For this review, take the finished solid that the model builds, in its own axes (mm). Round coordinates to 2 decimals unless told otherwise and drop trailing zeros. Order: outer loops, then holes, each group sorted by start corner. A loop starts at its lowest first (then second) coordinate and runs counter-clockwise, first axis right, second up. Notation, with made-up numbers: M -9.75,-11 L 45.25,-11 A25 cw 45.25,21 Z; hole C -23,-34.75 d11. An arc over 180 degrees is marked long. Put each result on its own line as item: value.
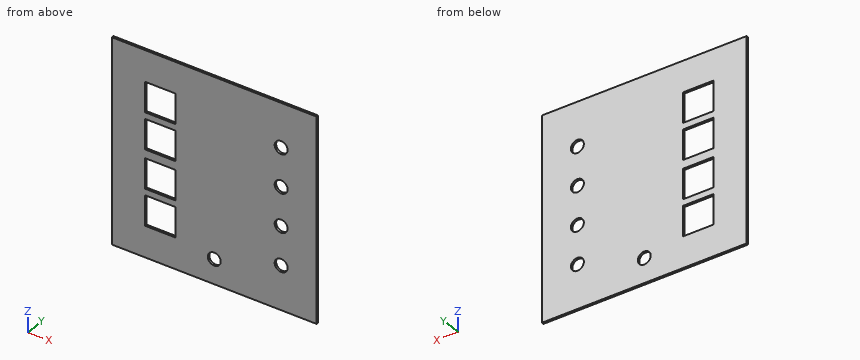
from build123d import *

# Parameters (mm, degrees)
SKETCH1_W           = 95
SKETCH1_H           = 95
BOSS_EXTRUDE1_DEPTH = 1
SKETCH2_R           = 3
SKETCH2_W           = 14
SKETCH2_H           = 14
CUT_EXTRUDE1_DEPTH  = 1


with BuildPart() as part:
    # Sketch1 → Boss-Extrude1 (new body)
    with BuildSketch(Plane(origin=(0, 0, 0), x_dir=(1, 0, 0), z_dir=(0, 1, 0))):
        with Locations((47.5, 47.5)):
            Rectangle(SKETCH1_W, SKETCH1_H)
    extrude(amount=BOSS_EXTRUDE1_DEPTH)

    # Sketch2 → Cut-Extrude1 (cut)
    with BuildSketch(Plane(origin=(0, 1, 0), x_dir=(1, 0, 0), z_dir=(0, 1, 0))):
        with Locations(Location((47.5, 83.5, 0), (0, 0, 270))):
            Circle(SKETCH2_R)
        with Locations(Location((78.5, 74.5, 0), (0, 0, 270))):
            Circle(SKETCH2_R)
        with Locations(Location((78.5, 56.5, 0), (0, 0, 270))):
            Circle(SKETCH2_R)
        with Locations(Location((78.5, 38.5, 0), (0, 0, 90))):
            Circle(SKETCH2_R)
        with Locations(Location((78.5, 20.5, 0), (0, 0, 90))):
            Circle(SKETCH2_R)
        with Locations((22.5, 56.5)):
            Rectangle(SKETCH2_W, SKETCH2_H)
        with Locations((22.5, 73.5)):
            Rectangle(SKETCH2_W, SKETCH2_H)
        with Locations((22.5, 21.5)):
            Rectangle(SKETCH2_W, SKETCH2_H)
        with Locations((22.5, 38.5)):
            Rectangle(SKETCH2_W, SKETCH2_H)
    extrude(amount=-CUT_EXTRUDE1_DEPTH, mode=Mode.SUBTRACT)


solid = part.part
(1) Add section B-B on x = 47.5. Give the boundary of the cut face in (y, z), then the cut area to 3 significant figures.
A:
outline: M 0,-95 L 1,-95 L 1,-86.5 L 0,-86.5 Z; M 0,-80.5 L 1,-80.5 L 1,0 L 0,0 Z
area: 89.0 mm2
(2) Add section A-A on z = -83.5. Give the boundary of the cut face in (x, y), then the cut area to 3 significant figures.
A:
outline: M 0,0 L 44.5,0 L 44.5,1 L 0,1 Z; M 50.5,0 L 95,0 L 95,1 L 50.5,1 Z
area: 89.0 mm2
(3) Add section C-C on z = -56.5. Give the boundary of the cut face in (x, y), then the cut area to 3 significant figures.
A:
outline: M 0,0 L 15.5,0 L 15.5,1 L 0,1 Z; M 29.5,0 L 75.5,0 L 75.5,1 L 29.5,1 Z; M 81.5,0 L 95,0 L 95,1 L 81.5,1 Z
area: 75.0 mm2
(4) Add section D-D on y = 0.6. State how many separate pieces and enclosed holes the cut face has, then the cut area to 3 significant figures.
A:
separate pieces: 1
enclosed holes: 9
area: 8,100 mm2
(5) To check wall thickness, follow L1, parallel to X at y = 0.8, z = -56.5; L2, parallel to X at y = 0.75, z = -61.5; L3, parallel to X at y = 0.65, z = -76. State the ranges of each line that lie inside material, in increasing order.
A:
L1: x = 0 to 15.5, 29.5 to 75.5, 81.5 to 95
L2: x = 0 to 15.5, 29.5 to 95
L3: x = 0 to 15.5, 29.5 to 75.9, 81.1 to 95
